Check sheet for the modelled part. Datum: model origin and axes. Units: mm. A direction names the side the tool comes from. Round coordinates to 2 decimals unless told otherwise and drop trailing zeros. Loops run counter-clockwise (first coordinate to the right, second up) from the corner with the lowest first, then second, coordinate; pieces in that order, holes last. Notation, with made-up numbers: (14.5, 59) - (35.5, 59) arc R27 ccw to (35.5, 91) - close; hole circle Ø3 at (10.25, 80). An arc over 180 degrees is marked (long way). Put each result on its own line as item: value. Start each with the question number.
Item 1: Tool access check on faces 1 (the flat face through (14, -9, 2)), 2 (the flat face through (12.99, 26, 2)). Record the directions out of +Z, -Z, +X, -X, +Y, -Y that give a thin tool (end or side, any length) a straight path to the whole face; none if there is none.
Item 2: Section check C-C, the plane z = 2.25. Record the cut outline in (x, y), and give its area (3 significant figures).
Item 3: Draft check along X on faces 3 (the cylindrical face through (9.54, 9.55, 2.46)), 4 (the cylindrical face through (-5.158, -3.955, 2.535)), 5 (the cylindrical face through (35.398, -6.148, 2.465)). Enter one of: pulls with the +X half, pulls with the -X half, needs draft (parallel to the pull), parting line crosses it, or undercut.
Item 4: Gauge pin test, flat ends, axial feed: pin 1 Ø1 at (y, z) = (-1.5, 1) entering from +X; pin 2 Ø3 at (y, z) = (29, 3.5) entering from -X; pin 3 Ø1 at (y, z) = (38, 3) entering from +X. Record the tip position at first contact, or that the pin passes through.
Item 5: Material ranges on line 1 along Y through (x, z) = (0, 2.85); line 2 along Y through (x, z) = (28, 1.25); line 3 along X through (y, z) = (3, 3.2), recorded low to high.
Item 6: Section check B-B, the plane x = 27.5. Record the cut outline in (y, z).
Item 7: Section check D-D, the plane y = 40.5. Record the cut outline in (x, z), and give its area (3 significant figures).
Item 8: Section check A-A, the plane y = 2. Record the cut outline in (x, z), and give its area (3 significant figures).
from build123d import *

# Parameters (mm, degrees)
EXTRUDE_1_OUTLINE_R   = 5
EXTRUDE_1_OUTLINE_R_2 = 1.9
EXTRUDE_1_OUTLINE_R_3 = 1.5
EXTRUDE_1_DEPTH       = 5
SKETCH_2_R            = 6.5
CUT_EXTRUDE_1_DEPTH   = 59.840235174


# Read off the part's stored shape, not the designer's step: 凸台-拉伸1
with BuildPart() as part:
    # 凸台-拉伸1 outline → 凸台-拉伸1 (new body)
    with BuildSketch(Plane.XY):
        with BuildLine():
            ThreePointArc((0, 9), (-8.999999903, -0.001320394), (0.002640787, -8.999999613))
            Line((0.002640787, -8.999999613), (28.4053363, -8.999999613))
            ThreePointArc((28.4053363, -8.999999613), (35.476644301, -6.070827227), (38.405336277, 1.000679757))
            Line((38.405336277, 1.000679757), (38.404522272, 12.982447292))
            ThreePointArc((38.404522272, 12.982447292), (38.33518919, 13.723699418), (38.129692452, 14.439264147))
            Line((38.129692452, 14.439264147), (28.440328317, 39.210942539))
            ThreePointArc((28.440328317, 39.210942539), (19.507207266, 44.158149523), (12.989987975, 36.296765334))
            Line((12.989987975, 36.296765334), (12.989987975, 15.549905346))
            ThreePointArc((12.989987975, 15.549905346), (12.853385476, 14.513488564), (12.452908102, 13.547860343))
            Line((12.452908102, 13.547860343), (10.978711226, 10.997954609))
            ThreePointArc((10.978711226, 10.997954609), (9.514768336, 9.535307706), (7.515791099, 8.999999613))
            Line((7.515791099, 8.999999613), (0, 9))
        make_face()
        Circle(EXTRUDE_1_OUTLINE_R, mode=Mode.SUBTRACT)
        with Locations((28.405336318, 0.999728686)):
            Circle(EXTRUDE_1_OUTLINE_R_2, mode=Mode.SUBTRACT)
        with Locations((28.405336318, 15.999728686)):
            Circle(EXTRUDE_1_OUTLINE_R_2, mode=Mode.SUBTRACT)
        with Locations((20.989987975, 36.296765334)):
            Circle(EXTRUDE_1_OUTLINE_R_3, mode=Mode.SUBTRACT)
    extrude(amount=EXTRUDE_1_DEPTH)

    # 草图2 → 切除-拉伸1 (cut, through all)
    with BuildSketch(Plane.XY.offset(5)):
        Circle(SKETCH_2_R)
    extrude(amount=-CUT_EXTRUDE_1_DEPTH, mode=Mode.SUBTRACT)


solid = part.part
Check result:
1. face 1: +Z, -Z, +X, -X, -Y
1. face 2: +Z, -Z, -X, +Y
2. outline: (0, -9) - (28.41, -9) arc R10 ccw to (38.41, 1) - (38.4, 12.98) arc R4 ccw to (38.13, 14.44) - (28.44, 39.21) arc R8 ccw to (12.99, 36.3) - (12.99, 15.55) arc R4 cw to (12.45, 13.55) - (10.98, 11) arc R4 cw to (7.52, 9) - (0, 9) arc R9 ccw to start; hole circle Ø13 at (0, 0); hole circle Ø3 at (20.99, 36.3); hole circle Ø3.8 at (28.41, 1); hole circle Ø3.8 at (28.41, 16)
2. area: 1,340 mm²
3. face 3: pulls with the -X half
3. face 4: undercut
3. face 5: pulls with the +X half
4. pin 1: x = 38.2
4. pin 2: x = 12.99
4. pin 3: x = 29.11
5. line 1: -9 to -6.5, 6.5 to 9
5. line 2: -9 to -0.86, 2.86 to 14.14, 17.86 to 40.15
5. line 3: -8.49 to -5.77, 5.77 to 38.41
6. outline: (-9, 0) - (-0.67, 0) - (-0.67, 5) - (-9, 5) - close; (2.67, 0) - (14.33, 0) - (14.33, 5) - (2.67, 5) - close; (17.67, 0) - (40.95, 0) - (40.95, 5) - (17.67, 5) - close
7. outline: (14.18, 0) - (27.8, 0) - (27.8, 5) - (14.18, 5) - close
7. area: 68.1 mm²
8. outline: (-8.77, 0) - (-6.18, 0) - (-6.18, 5) - (-8.77, 5) - close; (6.18, 0) - (26.79, 0) - (26.79, 5) - (6.18, 5) - close; (30.02, 0) - (38.41, 0) - (38.41, 5) - (30.02, 5) - close
8. area: 158 mm²
